Could you check a few things on this drawing? It's one solid part, dimensions in mm from its lowest x, y, z. Coordinates: 2 decimals unless noted, no trailing zeros. Loops run counter-clockwise (first coordinate to the right, second up) from the corner with the lowest first, then second, coordinate; pieces in that order, holes last. Notation, with made-up numbers: (-32.75, 17.25) -> (18.25, 17.25) arc R30 ccw to (18.25, 52.25) -> close; hole circle Ø7 at (-27.5, 21). An arc over 180 degrees is marked (long way). One line per question, with ' | ' between items.
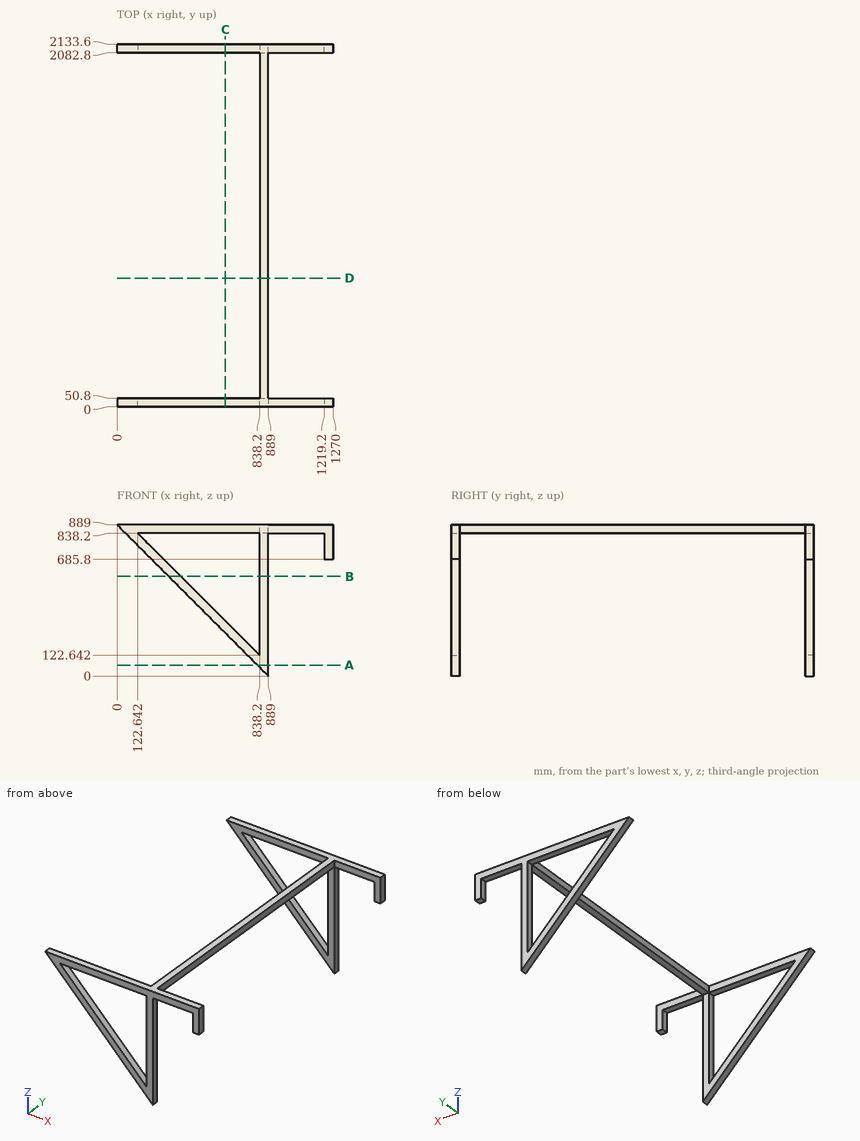
1) If we section it at A-A on z = 64.5: Please give me the cut outline in (x, y), and give its area (3 significant figures).
Data:
outline: (824.5, 0) -> (889, 0) -> (889, 50.8) -> (824.5, 50.8) -> close; (824.5, 2082.8) -> (889, 2082.8) -> (889, 2133.6) -> (824.5, 2133.6) -> close | area: 6,550 mm²
2) I'm going to push flat-ended pins straight in: pin 1 Ø15 at (y, z) = (33.5, 517) entering from +X; pin 2 Ø15 at (x, y) = (995.5, 26) entering from -Z; pin 3 Ø15 at (y, z) = (27, 620) entering from -X. Where does each tip first touch, or does it pass through?
Data:
pin 1: x = 889 | pin 2: z = 838.2 | pin 3: x = 261.5
3) If we section it at C-C on x = 636.5: Please give me the cut outline in (y, z), and give its area (3 significant figures).
Data:
outline: (0, 252.5) -> (50.8, 252.5) -> (50.8, 324.34) -> (0, 324.34) -> close; (0, 838.2) -> (50.8, 838.2) -> (50.8, 889) -> (0, 889) -> close; (2082.8, 252.5) -> (2133.6, 252.5) -> (2133.6, 324.34) -> (2082.8, 324.34) -> close; (2082.8, 838.2) -> (2133.6, 838.2) -> (2133.6, 889) -> (2082.8, 889) -> close | area: 12,500 mm²
4) If we section it at B-B on z = 586: Please give me the cut outline in (x, y).
Data:
outline: (303, 0) -> (374.84, 0) -> (374.84, 50.8) -> (303, 50.8) -> close; (303, 2082.8) -> (374.84, 2082.8) -> (374.84, 2133.6) -> (303, 2133.6) -> close; (838.2, 0) -> (889, 0) -> (889, 50.8) -> (838.2, 50.8) -> close; (838.2, 2082.8) -> (889, 2082.8) -> (889, 2133.6) -> (838.2, 2133.6) -> close
5) If we section it at D-D on y = 757: Please give me the cut outline in (x, z).
Data:
outline: (838.2, 838.2) -> (889, 838.2) -> (889, 889) -> (838.2, 889) -> close
6) I need wall thicknesses on line 1 along Y through (x, z) = (744, 216.5). Which ranges of the line are inside material? Lowest first, please. Write a range as from..to.
Data:
line 1: 0..50.8, 2082.8..2133.6
